Part model, mm, in its own coordinate system. A direction names the side the tool comes from. Coordinates: 2 decimals unless noted, no trailing zeros. Write each loop counter-clockwise with the first axis right and the second up, starting at its lowest first coordinate (ties: lowest second). Pieces come first, ordered by that corner, then holes. Notation, with made-up numbers: (40.25, 27.25) - (93.25, 27.25) arc R34 ccw to (93.25, 60.25) - close; hole circle Ø3 at (-20, -24.5). An arc over 180 degrees is marked (long way). Use a Markdown table: item, result.
```python
from build123d import *

# Parameters (mm, degrees)
SKETCH_1_R        = 14.5
SKETCH_1_R_2      = 12.5
EXTRUDE_1_DEPTH   = 15
EXTRUDE_START     = 10
SKETCH_1_3_W      = 220
SKETCH_1_3_H      = 100
SKETCH_1_3_R      = 12.5
EXTRUDE_1_2_DEPTH = 10
SKETCH_2_W        = 15
SKETCH_2_H        = 100
EXTRUDE_2_DEPTH   = 50
FILLET_1_R        = 5


with BuildPart() as part:
    # 草图1 → Extrude 1 (new body)
    with BuildSketch(Plane.XY):
        Circle(SKETCH_1_R)
        Circle(SKETCH_1_R_2, mode=Mode.SUBTRACT)
    extrude(amount=-EXTRUDE_1_DEPTH)

    # 草图1<3> → Extrude 1 2 (add)
    with BuildSketch(Plane.XY.offset(EXTRUDE_START)):
        Rectangle(SKETCH_1_3_W, SKETCH_1_3_H)
        Circle(SKETCH_1_3_R, mode=Mode.SUBTRACT)
    extrude(amount=-EXTRUDE_1_2_DEPTH)

    # 草图2 → 凸台-拉伸2 (add)
    with BuildSketch(Plane.XY.offset(10)):
        with Locations((-102.5, 0)):
            Rectangle(SKETCH_2_W, SKETCH_2_H)
        with Locations((102.5, 0)):
            Rectangle(SKETCH_2_W, SKETCH_2_H)
    extrude(amount=EXTRUDE_2_DEPTH)

    # 圆角1
    fillet_1_edges = [part.edges().sort_by_distance(p)[0] for p in [
        (-110, 0, 0),
        (110, 0, 0),
        (-95, 0, 10),
        (-102.5, -50, 60),
        (-102.5, 50, 60),
        (95, 0, 10),
        (102.5, 50, 60),
        (102.5, -50, 60),
    ]]
    fillet(fillet_1_edges, radius=FILLET_1_R)


solid = part.part
```
Item 1: Drill centre lines: probe 1 along Y at (x, z) = (0, -2); probe 2 along Y at (x, z) = (0, 3); probe 3 along Z at (x, y) = (78.5, -3). Where is each one in solid material? Low to high.
From the geometry:
| item | result |
|---|---|
| probe 1 | -14.5 to -12.5, 12.5 to 14.5 |
| probe 2 | -50 to -12.5, 12.5 to 50 |
| probe 3 | 0 to 10 |
Item 2: Band-saw the part on D-D, the plane y = -40.5. Give the cut face in (x, z).
From the geometry:
| item | result |
|---|---|
| outline | (-110, 5) arc R5 ccw to (-105, 0) - (105, 0) arc R5 ccw to (110, 5) - (110, 60) - (95, 60) - (95, 15) arc R5 cw to (90, 10) - (-90, 10) arc R5 cw to (-95, 15) - (-95, 60) - (-110, 60) - close |
Item 3: Band-saw the part on B-B, the plane y = 0. Give the cut face in (x, z), then the cut area to 3 significant figures.
From the geometry:
| item | result |
|---|---|
| outline | (-110, 5) arc R5 ccw to (-105, 0) - (-14.5, 0) - (-14.5, -15) - (-12.5, -15) - (-12.5, 10) - (-90, 10) arc R5 cw to (-95, 15) - (-95, 60) - (-110, 60) - close; (12.5, -15) - (14.5, -15) - (14.5, 0) - (105, 0) arc R5 ccw to (110, 5) - (110, 60) - (95, 60) - (95, 15) arc R5 cw to (90, 10) - (12.5, 10) - close |
| area | 3,510 mm^2 |
Item 4: Which spindle directions (+Z, -Z, +X, -X, +Y, -Y) get a long thin tool onto all of the face, cutting with end or side? Do faces 1 (the face through (6.691, -12.864, -7.395)), 2 (the face through (11.923, 3.755, -2.325)), 3 (the face through (95, -1, 37)). Say none if no direction does.
From the geometry:
| item | result |
|---|---|
| face 1 | -Z |
| face 2 | +Z, -Z |
| face 3 | +Z, +Y, -Y |
Item 5: Band-saw the part on A-A, the plane x = 0. Give the cut face in (y, z), then the cut area to 3 significant figures.
From the geometry:
| item | result |
|---|---|
| outline | (-50, 0) - (-14.5, 0) - (-14.5, -15) - (-12.5, -15) - (-12.5, 10) - (-50, 10) - close; (12.5, -15) - (14.5, -15) - (14.5, 0) - (50, 0) - (50, 10) - (12.5, 10) - close |
| area | 810 mm^2 |
Item 6: Two-plate mould, pull along X, no slides. Class faces 4 (the face through (-95, -1, 37)), 5 (the face through (102, 1, 60)), 6 (the face through (110, -1, 33)): pulls with the +X half, pulls with the -X half, needs draft (parallel to the pull), parting line crosses it, or undercut.
From the geometry:
| item | result |
|---|---|
| face 4 | undercut |
| face 5 | needs draft |
| face 6 | pulls with the +X half |
Item 7: Drop flat-ended pins along their axis: P1, Ø8, axis at x = 70, y = -29, coming from the -Z side; P2, Ø1, axis at x = 75.5, y = 19.5, coming from the +Z side; P3, Ø22.5, axis at x = 0, y = 0, coming from the -Z side. Give the stop position or say it passes through.
From the geometry:
| item | result |
|---|---|
| P1 | z = 0 |
| P2 | z = 10 |
| P3 | through |
Item 8: Band-saw the part on C-C, the plane z = 43.5. Give the cut face in (x, y), then the cut area to 3 significant figures.
From the geometry:
| item | result |
|---|---|
| outline | (-110, -50) - (-95, -50) - (-95, 50) - (-110, 50) - close; (95, -50) - (110, -50) - (110, 50) - (95, 50) - close |
| area | 3,000 mm^2 |
